```python
from build123d import *

# Parameters (mm, degrees)
SKETCH1_R           = 4.25
BASEHEAD_DEPTH      = 5
SKETCH2_R           = 2.5
BASEBODY_DEPTH      = 25
HEXAGONSOCKET_DEPTH = 2.5
TOPFILLET_R         = 0.625
CHAMFER1_SIZE       = 0.2


with BuildPart() as part:
    # Sketch1 → BaseHead (new body)
    with BuildSketch(Plane(origin=(0, 0, 0), x_dir=(0, 0, -1), z_dir=(1, 0, 0))):
        Circle(SKETCH1_R)
    extrude(amount=BASEHEAD_DEPTH)

    # Sketch2 → BaseBody (add)
    with BuildSketch(Plane(origin=(5, 0, 0), x_dir=(0, 0, -1), z_dir=(1, 0, 0))):
        Circle(SKETCH2_R)
    extrude(amount=BASEBODY_DEPTH)

    # Sketch3 → HexagonSocket (cut)
    with BuildSketch(Plane(origin=(0, 0, 0), x_dir=(0, 0, -1), z_dir=(1, 0, 0))):
        Polygon((2.309401077, 0), (1.154700538, 2), (-1.154700538, 2), (-2.309401077, 0), (-1.154700538, -2), (1.154700538, -2), align=None)
    extrude(amount=HEXAGONSOCKET_DEPTH, mode=Mode.SUBTRACT)

    # Sketch4 → Cut-Revolve1 (revolve, cut)
    with BuildSketch(Plane(origin=(-4.19613823, 0.75, 0), x_dir=(-1, 0, 0), z_dir=(0, 0, 1))):
        Polygon((-6.69613823, 2.75), (-7.850838768, 0.75), (-6.69613823, 0.75), align=None)
    revolve(axis=Axis((0.838992387, 0, 0), (-1, 0, 0)), mode=Mode.SUBTRACT)

    # TopFillet
    topfillet_edges = [part.edges().sort_by_distance(p)[0] for p in [
        (0, 0, 4.25),
    ]]
    fillet(topfillet_edges, radius=TOPFILLET_R)

    # Chamfer1
    chamfer1_edges = [part.edges().sort_by_distance(p)[0] for p in [
        (30, 0, 2.5),
    ]]
    chamfer(chamfer1_edges, length=CHAMFER1_SIZE)


solid = part.part
```
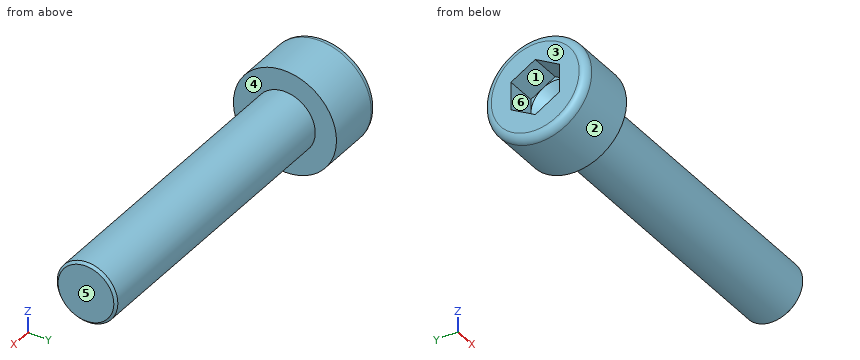
Model file for the job. Use its own axes, mm. Face numbers are marked on the shaded views. A direction names the side the tool comes from. Give positions to 0.01 mm unless a question says otherwise; leave off trailing zeros. Write each loop counter-clockwise with the first axis right and the second up, starting at its lowest first coordinate (ties: lowest second). Pieces come first, ordered by that corner, then holes. Notation, with made-up numbers: M 62.25,-40 L 89.25,-40 A17 ccw 89.25,-22 Z; hole C 63,50.25 d3. An arc over 180 degrees is marked long. Use a Markdown table: item, result.
1) Pull direction Y, two halves, no side cores. Call the marked faces 1, 2 and 3: +Y half, -Y half, draft (parallel to the pull), parting line (faces both ways), or undercut.
Responses:
| item | result |
|---|---|
| face 1 | undercut |
| face 2 | parting line |
| face 3 | draft |
2) Tool access for the marked faces 4, 5 and 6: list every direction of +Z, -Z, +X, -X, +Y, -Y with a clear straight run to the whole face (end or side of a thin tool).
Responses:
| item | result |
|---|---|
| face 4 | +X |
| face 5 | +Z, -Z, +X, +Y, -Y |
| face 6 | -X |
3) Pin check, flat tips, straight feed: pin 1 (5 mm diameter, centred on x = 16.5, z = -2.5, fed in from -Y); pin 2 (3 mm diameter, centred on x = 17.5, y = -1, fed in from +Z); pin 3 (2 mm diameter, centred on x = 5, z = 2.5, fed in from +Y). Stop position of each tip, or through.
Responses:
| item | result |
|---|---|
| pin 1 | stops at y = -2.5 |
| pin 2 | stops at z = 2.5 |
| pin 3 | stops at y = 3.98 |
4) Cut at A-A (x = 27). List the corners of the cut face in (y, z).
Responses:
| item | result |
|---|---|
| outline | C 0,0 d5 |
5) Drill centre lines: line 1 (Y direction, x = 9.25, z = -1.5); line 2 (X direction, y = 1.75, z = 2); line 3 (Z direction, x = 1.75, y = 1). Where is each one in solid material? Low to high. Write a range as from..to.
Responses:
| item | result |
|---|---|
| line 1 | y = -2..2 |
| line 2 | x = 0..5 |
| line 3 | z = -4.13..-1.73, 1.73..4.13 |
